Geometry: see drawing. Coordinates: mm, zero at the bounding-box minimum. A direction names the side the tool comes from. Give positions to 0.01 mm unless a question says otherwise; leave off trailing zeros. Write each loop counter-clockwise with the first axis right and the second up, starting at its lowest first coordinate (ties: lowest second). Pieces come first, ordered by that corner, then holes. Notation, with made-up numbers: M 73,55.5 L 106,55.5 A22 cw 106,79.5 Z; hole C -3.5,77 d3. An arc over 180 degrees is marked long. Answer as a JSON object with one key per item and string values. Group by question number.
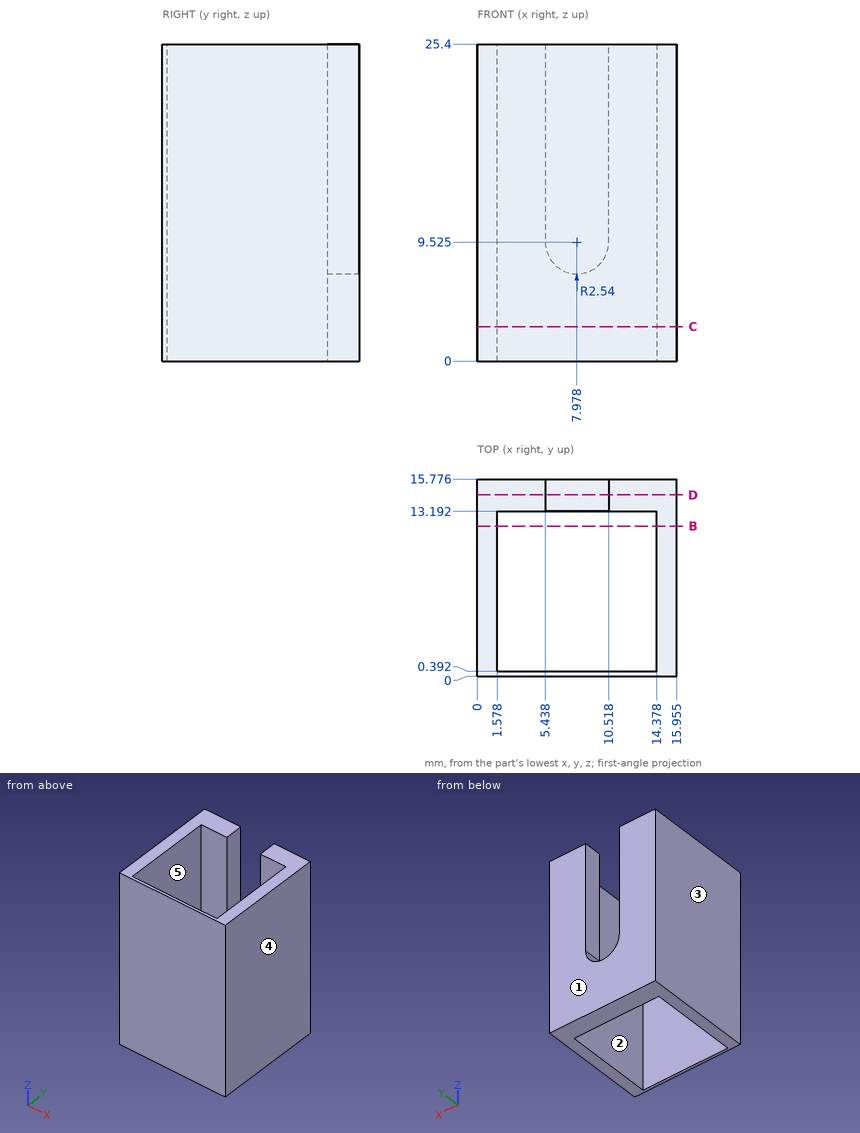
(1) Ray query, L1, parallel to X at y = 2.25, z = 5.75 (1 decimal); L2, parallel to Y at x = 12.25, z = 22.25 (1 decimal); L3, parallel to X at y = 13.25, z = 15.75 (1 decimal). Return the intervals inside material, ascending. Write a range as [from, to].
(2) Section D-D, the plane y = 14.5. Return loops of the section in (x, z) (1 decimal).
(3) Section C-C, the plane z = 2.75. Return loops of the section in (x, y) (1 decimal).
(4) Contact query for flat-ended pins moving along their axis: pin 1 Ø1.5 at (x, z) = (9.5, 9) entering from +Y; pin 2 Ø3 at (x, y) = (10.5, 10.5) entering from +Z. Output: stop coordinate, or through.
(5) Access query for the marked faces 4 and 5. Directions: +Z, -Z, +X, -X, +Y, -Y. A direction counts if a zero-diameter tool reaches every point of the face in a straight line with its end or side. Return the directions, or none.
(6) Pull-direction query (X, two-part tool) for the marked faces 1, 2 and 3; classes: pulls with the +X half, pulls with the -X half, needs draft (parallel to the pull), parting line crosses it, or undercut.
(7) Section B-B, the plane y = 12. Return loops of the section in (x, z) (1 decimal).
Reported:
{
 "1": {"L1": "x = [0, 1.6], [14.4, 16]", "L2": "y = [0, 0.4], [13.2, 15.8]", "L3": "x = [0, 5.4], [10.5, 16]"},
 "2": {"outline": "M 0,0 L 16,0 L 16,25.4 L 10.5,25.4 L 10.5,9.5 A2.5 cw 5.4,9.5 L 5.4,25.4 L 0,25.4 Z"},
 "3": {"outline": "M 0,0 L 16,0 L 16,15.8 L 0,15.8 Z; hole M 1.6,0.4 L 14.4,0.4 L 14.4,13.2 L 1.6,13.2 Z"},
 "4": {"pin 1": "stops at y = 0.39", "pin 2": "passes through"},
 "5": {"face 4": "+Z, -Z, +X, +Y, -Y", "face 5": "+Z, -Z"},
 "6": {"face 1": "needs draft", "face 2": "undercut", "face 3": "pulls with the -X half"},
 "7": {"outline": "M 0,0 L 1.6,0 L 1.6,25.4 L 0,25.4 Z; M 14.4,0 L 16,0 L 16,25.4 L 14.4,25.4 Z"}
}
